from build123d import *

# Parameters (mm, degrees)
SKETCH1_W           = 57
SKETCH1_H           = 33
BOSS_EXTRUDE1_DEPTH = 10
SKETCH3_R           = 3.35
CUT_EXTRUDE1_DEPTH  = 11
SKETCH4_R           = 3.35
CUT_EXTRUDE2_DEPTH  = 11
SKETCH10_R          = 3.35
CUT_EXTRUDE5_DEPTH  = 11
SKETCH12_R          = 3.35
CUT_EXTRUDE6_DEPTH  = 11
SKETCH16_W          = 57
SKETCH16_H          = 4
CUT_EXTRUDE7_DEPTH  = 4


with BuildPart() as part:
    # Sketch1 → Boss-Extrude1 (new body)
    with BuildSketch(Plane(origin=(0, 0, 0), x_dir=(1, 0, 0), z_dir=(0, 1, 0))):
        with Locations((28.5, 16.5)):
            Rectangle(SKETCH1_W, SKETCH1_H)
    extrude(amount=BOSS_EXTRUDE1_DEPTH)

    # Sketch3 → Cut-Extrude1 (cut, through all)
    with BuildSketch(Plane.XZ):
        with Locations((6, -6.5)):
            Circle(SKETCH3_R)
    extrude(amount=-CUT_EXTRUDE1_DEPTH, mode=Mode.SUBTRACT)

    # Sketch4 → Cut-Extrude2 (cut, through all)
    with BuildSketch(Plane.XZ):
        with Locations((51, -26.5)):
            Circle(SKETCH4_R)
    extrude(amount=-CUT_EXTRUDE2_DEPTH, mode=Mode.SUBTRACT)

    # Sketch10 → Cut-Extrude5 (cut, through all)
    with BuildSketch(Plane.XZ):
        with Locations((6, -26.5)):
            Circle(SKETCH10_R)
    extrude(amount=-CUT_EXTRUDE5_DEPTH, mode=Mode.SUBTRACT)

    # Sketch12 → Cut-Extrude6 (cut, through all)
    with BuildSketch(Plane.XZ):
        with Locations((51, -6.5)):
            Circle(SKETCH12_R)
    extrude(amount=-CUT_EXTRUDE6_DEPTH, mode=Mode.SUBTRACT)

    # Sketch16 → Cut-Extrude7 (cut)
    with BuildSketch(Plane(origin=(0, 10, 0), x_dir=(1, 0, 0), z_dir=(0, 1, 0))):
        with Locations((28.5, 16.5)):
            Rectangle(SKETCH16_W, SKETCH16_H)
    extrude(amount=-CUT_EXTRUDE7_DEPTH, mode=Mode.SUBTRACT)


solid = part.part
Check sheet for the modelled part. Datum: model origin and axes. Units: mm. A direction names the side the tool comes from. Round coordinates to 2 decimals unless told otherwise and drop trailing zeros. Loops run counter-clockwise (first coordinate to the right, second up) from the corner with the lowest first, then second, coordinate; pieces in that order, holes last. Notation, with made-up numbers: M 40.25,87 L 89.25,87 A19 ccw 89.25,103 Z; hole C 40,89 d2. An arc over 180 degrees is marked long. One line per item, written item: value.
(1) Depth check by flat-ended pin: pin 1 Ø5.5 at (x, z) = (51, -26.5) entering from +Y; pin 2 Ø1.2 at (x, z) = (29.5, -16.5) entering from +Y. Enter the tip coordinate at first touch or a pass-through.
Computed values:
pin 1: passes through
pin 2: stops at y = 6
(2) Access from +Z, -Z, +X, -X, +Y, -Y to the whole of each face (thin tool, end or side, straight path). Record for faces 4 (the face through (28, 8, -14.5)), 5 (the face through (9.195, 4.93, -5.494)).
Computed values:
face 4: +X, -X, +Y
face 5: +Y, -Y
(3) Sectioned sample at C-C, the plane y = 3.5. Record the cut outline in (x, z), then the cut area to 3 significant figures.
Computed values:
outline: M 0,-33 L 57,-33 L 57,0 L 0,0 Z; hole C 6,-26.5 d6.7; hole C 6,-6.5 d6.7; hole C 51,-26.5 d6.7; hole C 51,-6.5 d6.7
area: 1,740 mm^2
(4) Release check for a two-part mould opening along X. For faces 1 (the face through (54.195, 4.93, -25.494)), 2 (the face through (28, 10, -26)), 3 (the face through (57, 5, -16)) record: +X half, -X half, draft (parallel to the pull), parting line (faces both ways), or undercut.
Computed values:
face 1: undercut
face 2: draft
face 3: +X half
(5) Sectioned sample at B-B, the plane z = -26.5. Record the cut outline in (x, y).
Computed values:
outline: M 0,0 L 2.65,0 L 2.65,10 L 0,10 Z; M 9.35,0 L 47.65,0 L 47.65,10 L 9.35,10 Z; M 54.35,0 L 57,0 L 57,10 L 54.35,10 Z
(6) Thickness scan on line 1 (Z direction, x = 6, y = 7.25); line 2 (Z direction, x = 6, y = 3.5); line 3 (X direction, y = 2.25, z = -5). Record the ranges inside material, lowest first.
Computed values:
line 1: z = -33 to -29.85, -23.15 to -18.5, -14.5 to -9.85, -3.15 to 0
line 2: z = -33 to -29.85, -23.15 to -9.85, -3.15 to 0
line 3: x = 0 to 3, 9 to 48, 54 to 57
(7) Sectioned sample at D-D, the plane x = 19. Record the cut outline in (y, z).
Computed values:
outline: M 0,-33 L 10,-33 L 10,-18.5 L 6,-18.5 L 6,-14.5 L 10,-14.5 L 10,0 L 0,0 Z
(8) Sectioned sample at A-A, the plane x = 6. Record the cut outline in (y, z).
Computed values:
outline: M 0,-33 L 10,-33 L 10,-29.85 L 0,-29.85 Z; M 0,-23.15 L 10,-23.15 L 10,-18.5 L 6,-18.5 L 6,-14.5 L 10,-14.5 L 10,-9.85 L 0,-9.85 Z; M 0,-3.15 L 10,-3.15 L 10,0 L 0,0 Z
